Autodesk Inventor part; units mm, degrees
ref_plane "YZ Plane" through (0, 0, 0) normal (1, 0, 0) x (0, 1, 0)
ref_plane "XZ Plane" through (0, 0, 0) normal (0, 1, 0) x (-1, 0, 0)
ref_plane "XY Plane" through (0, 0, 0) normal (0, 0, 1) x (1, 0, 0)
sketch "Sketch1" plane through (0, 0, 0) normal (0, 0, 1) x (1, 0, 0)
  line L0 (-0.7124, 0.6699) -> (-6.35, 5.9705)
  line L1 (-6.35, 5.9705) -> (-103.1875, 0)
  line L2 (-102.9919, -6.35) -> (-5.9705, -6.35)
  line L3 (-5.9705, -6.35) -> (-0.6699, -0.7124)
  arc A0 (-103.1875, 0) -> (-102.9919, -6.35) centre (0, 0) ccw
  arc A1 (-0.7124, 0.6699) -> (-0.6699, -0.7124) centre (0, 0) ccw
  line L4 (0, 0) -> (-0.7124, 0.6699) construction
  line L5 (0, 0) -> (-0.6699, -0.7124) construction
  dimension "d0" = 103.1875
  dimension "d1" = 6.35
  dimension "d2" = 103.1875
  dimension "d3" = 6.35
  dimension "d7" = 1.9558
extrude "Extrusion1" add sketch "Sketch1" along normal blind 6.35
fillet "Fillet2" radius 3.81 2 edges at (-54.4812, -6.35, 6.35) (-54.7687, 2.9853, 6.35)
properties part number "Thrust_Support"
Design review of the part built by this model. Coordinates are the model's own, in mm. Coordinates: 2 decimals unless noted, no trailing zeros. Order: outer loops, then holes, each group sorted by start corner. A loop starts at its lowest first (then second) coordinate and runs counter-clockwise, first axis right, second up. Notation, with made-up numbers: M 5,-21.75 L 20,-21.75 A22 ccw 20,1.25 Z; hole C -29.5,22 d10. An arc over 180 degrees is marked long. Answer as a JSON object with one key per item and string values. Group by question number.
1) Add section C-C, the plane z = 5.25. Write out the cut boundary in (x, y).
2) Wall thickness on L1, parallel to Z at x = -49, y = -3.25; L2, parallel to Y at x = -75.5, z = 3.75; L3, parallel to Y at x = -28, z = 2.5: over which ranges is each line inside the solid? List them lowest first.
3) Add section B-B, the plane y = -5. Write out the cut boundary in (x, z), then the cut area to 3 significant figures.
4) For pin 1 (6 mm diameter, centred on x = -90.5, y = 2, fed in from +Z); pin 2 (1.5 mm diameter, centred on x = -29, y = 4, fed in from +Z), all flat-tipped, find the tip position at first contact; note any pin that passes through.
5) Add section A-A, the plane z = 1. Write out the cut boundary in (x, y), then the cut area to 3 significant figures.
Computed values:
{
 "1": {"outline": "M -103.18,-1.13 A103.16 ccw -103.06,-5.22 L -4.91,-5.22 L -0.67,-0.71 A0.98 cw -0.71,0.67 L -5.22,4.91 Z"},
 "2": {"L1": "z = 0 to 6.28", "L2": "y = -6.15 to 1.51", "L3": "y = -6.35 to 4.64"},
 "3": {"outline": "M -103.07,0 L -4.7,0 L -4.7,5.45 L -103.07,5.45 Z", "area": "536 mm^2"},
 "4": {"pin 1": "stops at z = 5.77", "pin 2": "stops at z = 5.43"},
 "5": {"outline": "M -103.19,0 A103.16 ccw -102.99,-6.35 L -5.97,-6.35 L -0.67,-0.71 A0.98 cw -0.71,0.67 L -6.35,5.97 Z", "area": "943 mm^2"}
}
